Can you work these out from the model? Positions are in its coordinate system, mm. Face numbers are marked on the shaded views. A direction names the side the tool comes from. Give positions to 0.01 mm unless a question says otherwise; leave off trailing zeros. Order: outer loops, then holes, each group sorted by start corner. A loop starts at its lowest first (then second) coordinate and runs counter-clockwise, first axis right, second up. Notation, with made-up numbers: M 25,-9 L 46,-9 A14 ccw 46,-4 Z; hole C 55,26 d7. An arc over 180 degrees is marked long. Answer as a JSON object with one key per item and string values.
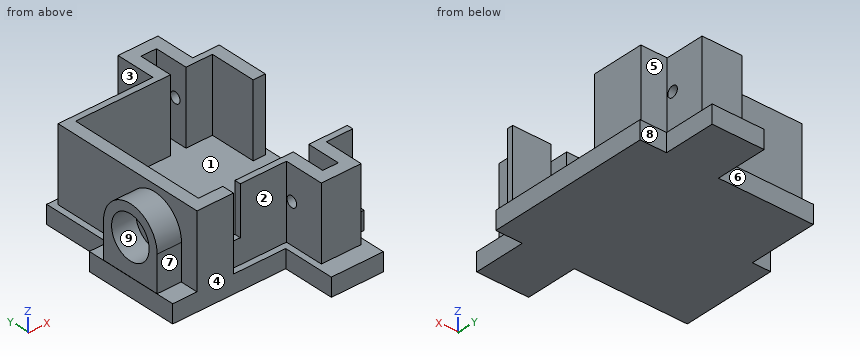
Autodesk Inventor part; units mm, degrees
ref_plane "Work Plane1" through (-15.1369, -12.3631, 5) normal (-1, 0, 0) x (0, 0, 1)
ref_plane "Work Plane2" through (0.4631, -17.8631, 14) normal (-1, 0, 0) x (0, 0, 1)
ref_plane "YZ Plane" through (0, 0, 0) normal (1, 0, 0) x (0, 1, 0)
sketch "Sketch1" plane through (0, 0, 0) normal (0, 0, 1) x (1, 0, 0)
  line L0 (-20, -23) -> (20, -23)
  line L1 (20, -23) -> (20, 23)
  line L2 (20, 23) -> (-20, 23)
  line L3 (-20, 23) -> (-20, -23)
  line L4 (-20, -23) -> (20, 23) construction
  line L5 (20, -23) -> (-20, 23) construction
  point P0 (0, 0)
  dimension "Szelesseg" = 40
  dimension "Magassag" = 46
extrude "Extrusion1" add sketch "Sketch1" along normal blind 3
sketch "Sketch12" plane through (0, 0, 3) normal (0, 0, 1) x (1, 0, 0)
  line L0 (9.3631, -11.3631) -> (5.0131, -11.3631)
  line L1 (5.0131, -11.3631) -> (5.0131, -16.8631)
  line L2 (2.4631, -15.3356) -> (2.4631, -11.3631)
  line L3 (-13.1369, -11.3631) -> (-13.1369, 11.5369)
  line L4 (-13.1369, 11.5369) -> (2.4631, 11.5369)
  line L5 (2.4631, 11.5369) -> (2.4631, 17.0369)
  line L6 (2.4631, 17.0369) -> (5.0131, 17.0369)
  line L7 (5.0131, 17.0369) -> (5.0131, 11.5369)
  line L8 (5.0131, 11.5369) -> (9.3631, 11.5369)
  line L9 (9.3631, 11.5369) -> (9.3631, 3.9369)
  line L10 (7.0131, -12.3631) -> (7.0131, -18.8631)
  line L11 (7.0131, -18.8631) -> (0.4631, -18.8631)
  line L12 (0.4631, -18.8631) -> (0.4631, -12.3631)
  line L13 (-15.1369, -13.3631) -> (-15.1369, 12.5369)
  line L14 (-15.1369, 12.5369) -> (0.4631, 12.5369)
  line L15 (0.4631, 12.5369) -> (0.4631, 19.0369)
  line L16 (0.4631, 19.0369) -> (7.0131, 19.0369)
  line L17 (7.0131, 19.0369) -> (7.0131, 12.5369)
  line L18 (7.0131, 12.5369) -> (11.3631, 12.5369)
  line L19 (11.3631, 12.5369) -> (11.3631, 5.6471)
  line L20 (7.0131, -12.3631) -> (13.6631, -12.3631)
  line L21 (13.6631, -12.3631) -> (13.6631, -11.3631)
  line L22 (13.6631, -11.3631) -> (9.3631, -11.3631)
  line L23 (-9.1369, -13.3631) -> (-9.1369, -11.3631)
  line L24 (-7.1369, -12.3631) -> (-7.1369, -11.3631)
  line L25 (0.4631, -12.3631) -> (-7.1369, -12.3631)
  line L26 (-9.1369, -13.3631) -> (-15.1369, -13.3631)
  line L27 (2.4631, -11.3631) -> (-7.1369, -11.3631)
  line L28 (-9.1369, -11.3631) -> (-13.1369, -11.3631)
  line L29 (-18.3631, -21.3631) -> (-18.3631, 21.3631)
  line L30 (18.3631, 21.3631) -> (18.3631, -21.3631)
  line L31 (18.3631, -21.3631) -> (-18.3631, -21.3631)
  line L32 (-18.3631, 21.3631) -> (18.3631, 21.3631)
  line L33 (2.4631, -15.3356) -> (2.4631, -16.8631)
  line L34 (-16.127, -19.127) -> (16.127, -19.127)
  line L35 (2.4631, -16.8631) -> (5.0131, -16.8631)
  line L36 (11.3631, 5.6471) -> (11.3631, 3.9369)
  line L37 (11.3631, 3.9369) -> (9.3631, 3.9369)
  line L38 (-9.1369, -12.3631) -> (-7.1369, -12.3631)
  line L39 (-9.1369, -11.3631) -> (-7.1369, -11.3631)
  point P0 (19.6785, 0.2929)
  dimension "d83" = 22.5
  dimension "d85" = 2.55
  dimension "d86" = 2.55
  dimension "d87" = 15.6
  dimension "d88" = 15.6
  dimension "d89" = 4.35
  dimension "d90" = 4.35
  dimension "d91" = 7.6
  dimension "d92" = 5.5
  dimension "d95" = 22.9
  dimension "d97" = 2
  dimension "d98" = 2
  dimension "d99" = 2
  dimension "d100" = 2
  dimension "d101" = 2
  dimension "d102" = 2
  dimension "d103" = 4.3
  dimension "d105" = 2
  dimension "d106" = 1
  dimension "d107" = 1
  dimension "d109" = 1
  dimension "d110" = 4
  dimension "d111" = 2
  dimension "d112" = 2
  dimension "d113" = 1
  dimension "d114" = 22.9
  dimension "d125" = 2.5
  dimension "d130" = 4.7
  dimension "d132" = 9
  dimension "d133" = 5.5
  dimension "d139" = 2
extrude "Extrusion4" add sketch "Sketch12" along normal blind 12 contours L22 L21 L20 L10 L11 L12 L25 L24 L27 L2 L33 L35 L1 L0 | L24 L38 L23 L39 | L23 L26 L13 L14 L15 L16 L17 L18 L19 L36 L37 L9 L8 L7 L6 L5 L4 L3 L28
sketch "Sketch14" plane through (0, 0, 15) normal (0, 0, 1) x (1, 0, 0)
  line L0 (-9.1369, -12.3631) -> (0.4631, -12.3631)
  line L1 (-9.1369, -12.3631) -> (-9.1369, -11.3631)
  line L2 (-13.1369, -11.3631) -> (2.4631, -11.3631)
  line L3 (-7.1369, -11.3631) -> (-7.1369, -12.3631)
  point P0 (0, 0)
  dimension "d136" = 2
extrude "Extrusion5" cut sketch "Sketch14" against normal blind 8
sketch "Sketch17" plane through (7.0131, -18.8631, 3) normal (1, 0, 0) x (0, 0, -1)
  line L0 (0, 0) -> (-12, 0)
  line L1 (0, 7.5) -> (-12, 7.5)
  line L2 (0, 6.5) -> (-12, 6.5)
  line L3 (-12, 7.5) -> (-12, 30.4) construction
  line L4 (-12, 18.95) -> (0, 18.95) construction
  line L5 (0, 37.9) -> (-12, 37.9) construction
  line L6 (0, 31.4) -> (-12, 31.4) construction
  point P0 (3, 18.8631)
  point P1 (-6.5, 5.5)
  point P2 (-6.5, 32.4)
  dimension "d144" = 1
  dimension "d145" = 18.95
  dimension "d146" = 1
hole "Hole3" at (7.0131, -13.3631, 9.5) at (7.0131, 13.5369, 9.5) direction (-1, 0, 0) diameter 1.778 depth 8 tip angle 118
ref_plane "Work Plane1" through (-15.1369, -12.3631, 5) normal (-1, 0, 0) x (0, 0, 1)
sketch "Sketch18" plane through (-15.1369, -12.3631, 5) normal (-1, 0, 0) x (0, 0, 1)
  line L0 (10, 0) -> (0, 0)
  line L1 (-2, -9) -> (-2, 33.7262)
  circle A0 centre (3.9, 6.9) radius 3.5
  circle A1 centre (3.9, 6.9) radius 5
  point P0 (-5, 12.3631)
  point P1 (9, 0)
  dimension "d156" = 6.9
  dimension "d157" = 5.9
  dimension "d158" = 7
  dimension "d159" = 10
extrude "Extrusion6" add sketch "Sketch18" along normal blind 4
sketch "Sketch20" plane through (0, 0, 3) normal (0, 0, 1) x (1, 0, 0)
  point P0 (0, 0)
ref_plane "Work Plane2" through (0.4631, -17.8631, 14) normal (-1, 0, 0) x (0, 0, 1)
sketch "Sketch21" plane through (0.4631, -17.8631, 14) normal (-1, 0, 0) x (0, 0, 1)
  line L0 (-11, -3.5) -> (-11, 39.2262)
  arc A0 (-5.389, 4.5) -> (-3.611, 4.5) centre (-4.5, 4.5) ccw
  line L1 (0, 5.5) -> (-11, 5.5)
  point P0 (-14, 17.8631)
  point P1 (-9, 5.5)
  dimension "d164" = 6.5
  dimension "d165" = 1
sketch "Sketch22" plane through (-15.1369, -13.127, 3) normal (-1, 0, 0) x (0, 0, 1)
  circle A0 centre (5.9, 7.6639) radius 5
  line L0 (5.9, 12.6639) -> (0.0331, 12.6639)
  line L1 (5.9, 2.6639) -> (0.0331, 2.6639)
  line L2 (0.0331, 12.6639) -> (0.0331, 2.6639)
  line L3 (0, -0.2361) -> (0, 25.6639)
  point P0 (-3, 13.127)
  point P1 (0, 0)
  point P2 (0, 25.4279)
  point P3 (0, 0.7639)
  point P4 (0, 24.6639)
extrude "Extrusion7" add sketch "Sketch22" along normal blind 4 contours A0 L1 L2 L0
sketch "Sketch25" plane through (13.6631, -12.3631, 3) normal (1, 0, 0) x (0, 0, -1)
  line L0 (-12, 1) -> (-12, -4.5)
  line L1 (0, 1) -> (-12, 1)
  line L2 (-12, -0.0067) -> (0, -0.0067)
  line L3 (0, -0.0067) -> (0, 1)
  line L4 (0, 1) -> (-12, 1)
  line L5 (-12, 1) -> (-12, -0.0067)
  point P0 (3, 12.3631)
extrude "Extrusion8" cut sketch "Sketch25" against normal blind 2.3
sketch "Sketch26" plane through (0, 0, 3) normal (0, 0, 1) x (1, 0, 0)
  line L0 (-19.1369, -13.3631) -> (-19.1369, 2.1817)
  line L1 (-19.1369, -0.4631) -> (-19.1369, -10.4631)
  line L2 (-19.1369, 2.1817) -> (-16.1369, 2.1817)
  line L3 (-16.1369, 2.1817) -> (-16.1369, 13.5369)
  line L4 (-16.1369, 13.5369) -> (-0.5369, 13.5369)
  line L5 (-0.5369, 13.5369) -> (-0.5369, 22.0369)
  line L6 (-0.5369, 22.0369) -> (8.0131, 22.0369)
  line L7 (8.0131, 22.0369) -> (8.0131, 13.5369)
  line L8 (8.0131, 13.5369) -> (12.3631, 13.5369)
  line L9 (12.3631, 13.5369) -> (12.3631, -13.3631)
  line L10 (12.3631, -13.3631) -> (8.0131, -13.3631)
  line L11 (8.0131, -13.3631) -> (8.0131, -21.8631)
  line L12 (8.0131, -21.8631) -> (-0.5369, -21.8631)
  line L13 (-0.5369, -21.8631) -> (-0.5369, -13.3631)
  line L14 (-0.5369, -13.3631) -> (-19.1369, -13.3631)
  line L15 (-15.1369, -13.3631) -> (-15.1369, 12.5369)
  line L16 (0.4631, 12.5369) -> (-15.1369, 12.5369)
  line L17 (0.4631, 19.0369) -> (0.4631, 12.5369)
  line L18 (7.0131, 19.0369) -> (0.4631, 19.0369)
  line L19 (7.0131, 12.5369) -> (7.0131, 19.0369)
  line L20 (11.3631, 3.9369) -> (11.3631, 12.5369)
  line L21 (7.0131, -12.3631) -> (11.3631, -12.3631)
  line L22 (7.0131, -12.3631) -> (7.0131, -18.8631)
  line L23 (0.4631, -18.8631) -> (7.0131, -18.8631)
  line L24 (-7.1369, -12.3631) -> (0.4631, -12.3631)
  line L25 (-20, -23) -> (20, -23)
  line L26 (-20, -23) -> (20, -23)
  line L27 (20, -23) -> (20, 23)
  line L28 (20, 23) -> (-20, 23)
  line L29 (-20, 23) -> (-20, -23)
  point P0 (0, 0)
  dimension "d177" = 1
  dimension "d178" = 1
  dimension "d179" = 1
  dimension "d180" = 3
  dimension "d181" = 1
  dimension "d182" = 1
  dimension "d183" = 1
  dimension "d184" = 1
  dimension "d185" = 3
  dimension "d186" = 1
  dimension "d187" = 4
  dimension "d188" = 3
extrude "Extrusion9" cut sketch "Sketch26" against normal blind 10
sketch "Sketch27" plane through (0, 0, 3) normal (0, 0, 1) x (1, 0, 0)
  line L0 (-0.5369, 22.0369) -> (-0.5369, 13.5369)
  line L1 (8.0131, 22.0369) -> (-0.5369, 22.0369)
  line L2 (-0.5369, 19.0369) -> (8.0131, 19.0369)
  line L3 (8.0131, 19.0369) -> (8.0131, 22.0369)
  line L4 (8.0131, 22.0369) -> (-0.5369, 22.0369)
  line L5 (-0.5369, 22.0369) -> (-0.5369, 19.0369)
  line L6 (-0.5369, -21.8631) -> (-0.5369, -13.3631)
  line L7 (8.0131, -21.8631) -> (8.0131, -13.3631)
  line L8 (-0.5369, -21.8631) -> (8.0131, -21.8631)
  line L9 (8.0131, -21.8631) -> (8.0131, -18.8631)
  line L10 (8.0131, -18.8631) -> (-0.5369, -18.8631)
  line L11 (-0.5369, -18.8631) -> (-0.5369, -21.8631)
  point P0 (0, 0)
equation "\"d86\" = d85"
equation "\"d90\" = d89"
equation "\"d95\" = d82"
equation "\"d9\" = 0.5 * d10"
equation "\"d12\" = d11"
equation "\"d13\" = d11"
equation "\"d14\" = d11"
equation "\"d93\" = d92"
properties part number "Hip_rotation_temp"
1) Thinking about a two-plate mould opening in X: for the marked faces 1, 2, 3 and 4, which applies, pulls with the +X half, pulls with the -X half, needs draft (parallel to the pull), parting line crosses it, or undercut?
Results found:
{"face 1": "undercut", "face 2": "undercut", "face 3": "pulls with the -X half", "face 4": "needs draft"}
2) I need wall thicknesses on L1, parallel to Y at x = 1.85, z = 9.5; L2, parallel to X at y = -12, z = 8; L3, parallel to Y at x = 1, z = 8.5. Which ranges of each line are inside material? Lowest first, please.
Results found:
{"L1": "y = -18.86 to -14.25, -12.47 to -11.36, 11.54 to 12.65, 14.43 to 19.04", "L2": "x = -15.14 to -9.14, -7.14 to 2.46, 5.01 to 11.36", "L3": "y = -18.86 to -11.36, 11.54 to 19.04"}
3) For the marked faces 5, 6, 7, 8 and 9, which set-ups out of +Z, -Z, +X, -X, +Y, -Y let a thin tool reach every point of the face, with its end or its side?
Results found:
{"face 5": "+Z, +X, +Y", "face 6": "+Z, -Z, -X, +Y", "face 7": "+Z, -X, -Y", "face 8": "+Z, -Z, +X, +Y", "face 9": "-X"}
4) I want a section at B-B on x = 3. Write out the boundary of the cut face in (y, z), and give its area (3 significant figures).
Results found:
{"outline": "M -21.86,0 L 22.04,0 L 22.04,3 L 19.04,3 L 19.04,15 L 17.04,15 L 17.04,3 L -16.86,3 L -16.86,15 L -18.86,15 L -18.86,3 L -21.86,3 Z", "area": "180 mm²"}
5) I'm going to push flat-ended pins straight in: pin 1 Ø4.5 at (y, z) = (14, 9) entering from -X; pin 2 Ø3 at (x, y) = (5.5, -10.5) entering from -Z; pin 3 Ø1.5 at (x, z) = (-18, 1.5) entering from +Y; pin 4 Ø1.3 at (x, z) = (8, 10.5) entering from -Y. Where does each tip first touch, or does it pass through?
Results found:
{"pin 1": "stops at x = -15.14", "pin 2": "stops at z = 0", "pin 3": "stops at y = 2.18", "pin 4": "stops at y = -12.36"}
6) I want a section at D-D on z = 9.5. Count the separate pieces of the cut face and the enclosed holes in it, and give its area (3 significant figures).
Results found:
{"separate pieces": "6", "enclosed holes": "0", "area": "173 mm²"}
